The listing builds one solid part. Answer for the finished solid, in the listing's coordinates (mm). A direction names the side the tool comes from. Coordinates: 2 decimals unless noted, no trailing zeros. Write each loop counter-clockwise with the first axis right and the second up, starting at its lowest first coordinate (ties: lowest second). Pieces come first, ordered by that corner, then holes. Notation, with made-up numbers: M 17,69 L 27,69 A12 ccw 27,81 Z; hole C -12,68 d11. An arc over 180 degrees is marked long. Answer as CSV lines item,"result".
```python
from build123d import *

# Parameters (mm, degrees)
SKETCH1_R                = 1.6129
BOSS_EXTRUDE1_DEPTH      = 2.42062
SKETCH2_R                = 3.2258
BOSS_EXTRUDE2_DEPTH      = 1.6129
BOSS_EXTRUDE2_DEPTH_BACK = 1.5748
SKETCH3_R                = 2.42062
CUT_EXTRUDE1_DEPTH       = 2.42062


with BuildPart() as part:
    # Sketch1 → Boss-Extrude1 (new body)
    with BuildSketch(Plane.XY):
        with BuildLine():
            Line((-8.0772, -5.12826), (8.0772, -5.12826))
            ThreePointArc((8.0772, -5.12826), (9.567321834, -4.13259847), (9.217705328, -2.374880273))
            Line((9.217705328, -2.374880273), (3.421515983, 3.421439181))
            ThreePointArc((3.421515983, 3.421439181), (0, 4.8387), (-3.421515983, 3.421439181))
            Line((-3.421515983, 3.421439181), (-9.217705328, -2.374880273))
            ThreePointArc((-9.217705328, -2.374880273), (-9.567321834, -4.13259847), (-8.0772, -5.12826))
        make_face()
        Circle(SKETCH1_R, mode=Mode.SUBTRACT)
    extrude(amount=-BOSS_EXTRUDE1_DEPTH)

    # Sketch2 → Boss-Extrude2 (add, two sides)
    with BuildSketch(Plane.XZ.offset(5.12826)) as boss_extrude2_sk:
        with Locations((0, 2.82194)):
            Circle(SKETCH2_R)
    extrude(amount=BOSS_EXTRUDE2_DEPTH)
    extrude(boss_extrude2_sk.sketch, amount=-BOSS_EXTRUDE2_DEPTH_BACK)

    # Sketch3 → Cut-Extrude1 (cut)
    with BuildSketch(Plane.XZ.offset(6.74116)):
        with Locations((0, 2.82194)):
            Circle(SKETCH3_R)
    extrude(amount=-CUT_EXTRUDE1_DEPTH, mode=Mode.SUBTRACT)


solid = part.part
```
Q1. For faces 4 (the cylindrical face through (-0.525, -5.548, 0.459)), 5 (the cylindrical face through (0.05, 4.84, -1.19)), determine the directions among +Z, -Z, +X, -X, +Y, -Y from which every point of the face is accessible in a straight line to the end or side of a thin tool.
Output:
face 4,"-Y"
face 5,"+Z, -Z, +Y"
Q2. Find section B-B (z = -1). Give the vertices of the cut face in (x, y).
Output:
outline,"M -9.22,-2.37 A1.61 ccw -8.08,-5.13 L 8.08,-5.13 A1.61 ccw 9.22,-2.37 L 3.42,3.42 A4.84 ccw -3.42,3.42 Z; hole C 0,0 d3.23"
Q3. Find section A-A (x = 0). Give the vertices of the cut face in (y, z).
Output:
outline,"M -6.74,-0.4 L -5.13,-0.4 L -5.13,-2.42 L -1.61,-2.42 L -1.61,0 L -3.55,0 L -3.55,6.05 L -6.74,6.05 L -6.74,5.24 L -4.32,5.24 L -4.32,0.4 L -6.74,0.4 Z; M 1.61,-2.42 L 4.84,-2.42 L 4.84,0 L 1.61,0 Z"
Q4. Flat-ended cylindrical pins translate along their axes: pin 1 Ø3 at (x, z) = (6, 1) entering from -Y; pin 2 Ø4 at (x, y) = (3, 0) entering from +Z; pin 3 Ø4.5 at (x, z) = (0, 2.82) entering from -Y. Find the tip coordinate at first contact, or state that the pin passes through.
Output:
pin 1,"y = -5.13"
pin 2,"z = 0"
pin 3,"y = -4.32"
Q5. The mould has two halves that part along X. Classify faces 1 (the flat face through (0, -3.553, 3)), 2 (the cylindrical face through (9.557, -4.157, -1.193)), 3 (the flat face through (0, -4.321, 3)): pulls with the +X half, pulls with the -X half, needs draft (parallel to the pull), parting line crosses it, or undercut.
Output:
face 1,"needs draft"
face 2,"pulls with the +X half"
face 3,"undercut"
Q6. Find section C-C (y = 0). Give the vertices of the cut face in (x, z), and give its area (3 significant figures).
Output:
outline,"M -6.84,-2.42 L -1.61,-2.42 L -1.61,0 L -6.84,0 Z; M 1.61,-2.42 L 6.84,-2.42 L 6.84,0 L 1.61,0 Z"
area,"25.3 mm2"
Q7. Find section D-D (y = -4.75). Give the vertices of the cut face in (x, z), and give its area (3 significant figures).
Output:
outline,"M -9.12,-2.42 L 9.12,-2.42 L 9.12,0 L 1.56,0 A3.23 ccw long -1.56,0 L -9.12,0 Z; hole C 0,2.82 d4.84"
area,"57.6 mm2"
Q8. Straight lines are drawn through the part: line 1 (Y direction, x = 0, z = -1.8); line 2 (Z direction, x = 0, y = -5.75); line 3 (Y direction, x = -0.25, z = 4.75). For each, find the intervals that lie inside material, in ascending order.
Output:
line 1,"-5.13 to -1.61, 1.61 to 4.84"
line 2,"-0.4 to 0.4, 5.24 to 6.05"
line 3,"-4.32 to -3.55"
